Model file for the job. Use its own axes, mm. Face numbers are marked on the shaded views. A direction names the side the tool comes from. Coordinates: 2 decimals unless noted, no trailing zeros. Order: outer loops, then holes, each group sorted by start corner. A loop starts at its lowest first (then second) coordinate and runs counter-clockwise, first axis right, second up.
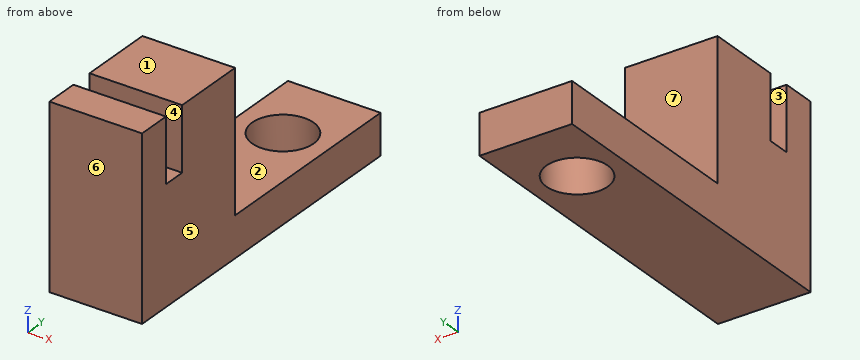
Autodesk Inventor part; units mm, degrees
ref_plane "YZ Plane" through (0, 0, 0) normal (1, 0, 0) x (0, 1, 0)
ref_plane "XZ Plane" through (0, 0, 0) normal (0, 1, 0) x (-1, 0, 0)
ref_plane "XY Plane" through (0, 0, 0) normal (0, 0, 1) x (1, 0, 0)
sketch "Sketch2" plane through (0, 0, 0) normal (1, 0, 0) x (0, 1, 0)
  line L0 (-8.2712, 6.008) -> (-8.2712, 0.508)
  line L1 (-8.2712, 0.508) -> (-10.2712, 0.508)
  line L2 (-10.2712, 0.508) -> (-10.2712, 6.008)
  line L3 (-10.2712, 6.008) -> (-13.2312, 6.008)
  line L4 (-13.2312, 6.008) -> (-13.2312, -9.492)
  line L5 (-13.2312, -9.492) -> (16.2688, -9.492)
  line L6 (16.2688, -5.992) -> (-1.7312, -5.992)
  line L7 (-1.7312, -5.992) -> (-1.7312, 6.008)
  line L8 (16.2688, -9.492) -> (16.2688, -5.992)
  line L9 (-1.7312, 6.008) -> (-8.2712, 6.008)
  point P0 (0, 0)
  dimension "d2" = 2
  dimension "d3" = 5.5
  dimension "d4" = 15.5
  dimension "d9" = 12
  dimension "d10" = 29.5
  dimension "d11" = 24.54
  dimension "d12" = 18
  dimension "d22" = 3.5
extrude "Extrusion1" add sketch "Sketch2" along normal blind 8
sketch "Sketch3" plane through (0, -1.7312, -5.992) normal (0, 0, 1) x (1, 0, 0)
  line L0 (0, 18) -> (8, 18)
  line L1 (0, 0) -> (0, 18)
  point P0 (0, 1.7312)
  point P1 (4, 11.65)
  dimension "d13" = 6.35
  dimension "d14" = 4
hole "Hole1" at (4, 9.9188, -5.992) direction (0, 0, -1) diameter 5.3 depth 8 tip angle 118
properties part number "grip1"
Q1. Mould opens along Y. For the marked faces 4, 5, 6 and 7 say: pulls with the +Y half, pulls with the -Y half, needs draft (parallel to the pull), parting line crosses it, or undercut.
Established:
face 4: undercut
face 5: needs draft
face 6: pulls with the -Y half
face 7: pulls with the +Y half
Q2. Cut at B-B, the plane z = 1. List the corners of the cut face in (x, y), plus the area to 3 significant figures.
Established:
outline: (0, -13.23) - (8, -13.23) - (8, -10.27) - (0, -10.27) - close; (0, -8.27) - (8, -8.27) - (8, -1.73) - (0, -1.73) - close
area: 76.0 mm2
Q3. Cut at C-C, the plane x = 7.5. List the corners of the cut face in (y, z), plus the area to 3 significant figures.
Established:
outline: (-13.23, -9.49) - (16.27, -9.49) - (16.27, -5.99) - (-1.73, -5.99) - (-1.73, 6.01) - (-8.27, 6.01) - (-8.27, 0.51) - (-10.27, 0.51) - (-10.27, 6.01) - (-13.23, 6.01) - close
area: 230 mm2
Q4. Cut at A-A, the plane x = 4. List the corners of the cut face in (y, z).
Established:
outline: (-13.23, -9.49) - (7.27, -9.49) - (7.27, -5.99) - (-1.73, -5.99) - (-1.73, 6.01) - (-8.27, 6.01) - (-8.27, 0.51) - (-10.27, 0.51) - (-10.27, 6.01) - (-13.23, 6.01) - close; (12.57, -9.49) - (16.27, -9.49) - (16.27, -5.99) - (12.57, -5.99) - close
Q5. Drop flat-ended pins along their axis: P1, Ø4, axis at x = 4, y = 8, coming from the +Z side; P2, Ø5, axis at y = 1.5, z = 1, coming from the -X side; P3, Ø4, axis at x = 7, z = 3, coming from the +Y side. Give the stop position or say it passes through.
Established:
P1: stops at z = -5.99
P2: passes through
P3: stops at y = -1.73
Q6. Which spindle directions (+Z, -Z, +X, -X, +Y, -Y) get a long thin tool onto all of the face, cutting with end or side? Do the marked faces 1, 2 and 3. Say none if no direction does.
Established:
face 1: +Z, +X, -X, +Y, -Y
face 2: +Z, +X, -X, +Y
face 3: +Z, +X, -X
Q7. Probe line 1 (Y direction, x = 4, z = -6.7); line 2 (Y direction, x = 6.5, z = 1); line 3 (Z direction, x = 4, y = -10). List the from-to ranges inside material, lowest first.
Established:
line 1: y = -13.23 to 7.27, 12.57 to 16.27
line 2: y = -13.23 to -10.27, -8.27 to -1.73
line 3: z = -9.49 to 0.51
Q8. Cut at D-D, the plane y = 12.25. List the corners of the cut face in (x, z).
Established:
outline: (0, -9.49) - (2.74, -9.49) - (2.74, -5.99) - (0, -5.99) - close; (5.26, -9.49) - (8, -9.49) - (8, -5.99) - (5.26, -5.99) - close
